The listing builds one solid part. Answer for the finished solid, in the listing's coordinates (mm). Face numbers are marked on the shaded views. A direction names the side the tool comes from. Round coordinates to 2 decimals unless told otherwise and drop trailing zeros. Loops run counter-clockwise (first coordinate to the right, second up) from the corner with the lowest first, then second, coordinate; pieces in that order, holes last. Notation, with made-up numbers: M 48.5,32 L 59.5,32 A11 cw 59.5,51 Z; hole C 76.5,-29.5 d7. An arc over 180 degrees is marked long. Put each result on its own line as item: value. Start each with the question number.
(1) Determine the mould class of the marked faces 1, 2 and 3 for opening direction Z: released by +Z, released by -Z, zero draft, split by the parting line, or undercut.
(2) Straight lines are drawn through the part: line 1 (X direction, y = 10, z = -16); line 2 (X direction, y = 12.5, z = -173.5); line 3 (Z direction, x = -100, y = 23). For each, find the intervals that lie inside material, in ascending order.
(3) Section B-B, the plane z = -173 is taken. Determine the outline of the cut face in (x, y), then the cut area to 3 significant figures.
(4) Which of the six approach directions +Z, -Z, +X, -X, +Y, -Y give full straight-line access (tool end or side, diameter ignored) to the marked faces 4, 5 and 6?
(5) Section C-C, the plane y = 7 is taken. Determine the outline of the cut face in (x, z).
(6) Section A-A, the plane x = 100 is taken. Determine the outline of the cut face in (y, z).
(7) Flat-ended cylindrical pins translate along their axes: P1, Ø5.5, axis at x = 69.5, z = -112, coming from the +Y side; P2, Ø1.5, axis at y = 25.5, z = -79, coming from the +X side; P3, Ø12, axis at y = 23.5, z = -163.5, coming from the -X side; P4, Ø12, axis at x = -54.5, z = -112, coming from the -Y side. Find the tip coordinate at first contact, or state that the pin passes through.
(8) Section D-D, the plane x = 14 is taken. Determine the outline of the cut face in (y, z).
```python
from build123d import *

# Parameters (mm, degrees)
SKETCH1_R                   = 12
BOSS_EXTRUDE1_DEPTH         = 33
FILLET1_R                   = 10
M8_TAPPED_HOLE1_D           = 6.8
M8_TAPPED_HOLE1_DEPTH       = 33
M8_TAPPED_HOLE1_CSINK_D     = 8.05
M8_TAPPED_HOLE1_CSINK_ANGLE = 90
CUT_EXTRUDE1_REACH          = 35


with BuildPart() as part:
    # Sketch1 → Boss-Extrude1 (new body)
    with BuildSketch(Plane(origin=(0, 0, 0), x_dir=(1, 0, 0), z_dir=(0, 1, 0))):
        with BuildLine():
            Line((125, 0), (-125, 0))
            Line((-125, 0), (-125, 148.505102572))
            ThreePointArc((-125, 148.505102572), (-120.023162168, 201.706671295), (-68.377223398, 188))
            Line((-68.377223398, 188), (68.377223398, 188))
            ThreePointArc((68.377223398, 188), (120.023162168, 201.706671295), (125, 148.505102572))
            Line((125, 148.505102572), (125, 0))
        make_face()
        with Locations((-100, 173)):
            Circle(SKETCH1_R, mode=Mode.SUBTRACT)
        with Locations((100, 173)):
            Circle(SKETCH1_R, mode=Mode.SUBTRACT)
    extrude(amount=BOSS_EXTRUDE1_DEPTH)

    # Fillet1
    fillet1_edges = [part.edges().sort_by_distance(p)[0] for p in [
        (-125, 16.5, -148.505102572),
        (-68.377223398, 16.5, -188),
        (68.377223398, 16.5, -188),
        (125, 16.5, -148.505102572),
    ]]
    fillet(fillet1_edges, radius=FILLET1_R)

    # M8 Tapped Hole1
    with Locations(Plane(origin=(0, 33, 0), x_dir=(1, 0, 0), z_dir=(0, 1, 0))):
        with Locations((-69.5, 112), (69.5, 112), (69.5, 16), (-69.5, 16)):
            CounterSinkHole(M8_TAPPED_HOLE1_D / 2, M8_TAPPED_HOLE1_CSINK_D / 2, depth=M8_TAPPED_HOLE1_DEPTH, counter_sink_angle=M8_TAPPED_HOLE1_CSINK_ANGLE)

    # Sketch4 → Cut-Extrude1 (cut, up to next)
    with BuildSketch(Plane(origin=(0, 33, 0), x_dir=(1, 0, 0), z_dir=(0, 1, 0)), mode=Mode.PRIVATE) as cut_extrude1_sk1:
        with BuildLine():
            Line((-41.773055434, 78.602374467), (36.226944566, 78.602374467))
            ThreePointArc((36.226944566, 78.602374467), (51.226944566, 63.602374467), (36.226944566, 48.602374467))
            Line((36.226944566, 48.602374467), (-41.773055434, 48.602374467))
            ThreePointArc((-41.773055434, 48.602374467), (-56.773055434, 63.602374467), (-41.773055434, 78.602374467))
        make_face()
    cut_extrude1_tool1 = extrude(cut_extrude1_sk1.sketch, amount=-CUT_EXTRUDE1_REACH, mode=Mode.PRIVATE) & part.part
    add(cut_extrude1_tool1.solids().sort_by_distance((-2.773055, 33, -63.602374))[0], mode=Mode.SUBTRACT)


solid = part.part
```
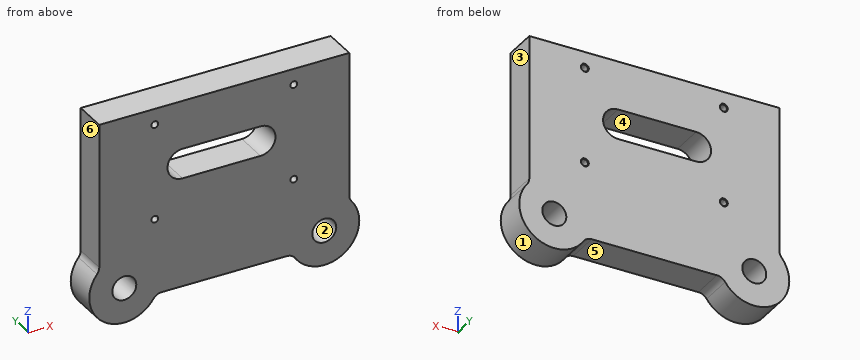
Recorded:
1. face 1: split by the parting line
1. face 2: undercut
1. face 3: zero draft
2. line 1: x = -125 to -72.9, -66.1 to 66.1, 72.9 to 125
2. line 2: x = -135 to -111.99, -88.01 to 88.01, 111.99 to 135
2. line 3: z = -208 to -185, -161 to 0
3. outline: M -135,0 L -112,0 L -112,33 L -135,33 Z; M -88,0 L 88,0 L 88,33 L -88,33 Z; M 112,0 L 135,0 L 135,33 L 112,33 Z
3. area: 7,330 mm²
4. face 4: +Y, -Y
4. face 5: -Z, +Y, -Y
4. face 6: +Z, -X, +Y, -Y
5. outline: M -127.22,-151 A35 ccw long -70.9,-192.44 A10 cw -62.58,-188 L 62.58,-188 A10 cw 70.9,-192.44 A35 ccw long 127.22,-151 A10 cw 125,-144.72 L 125,0 L -125,0 L -125,-144.72 A10 cw Z; hole C -100,-173 d24; hole C -69.5,-112 d6.8; hole C -69.5,-16 d6.8; hole M -41.77,-78.6 L 36.23,-78.6 A15 ccw 36.23,-48.6 L -41.77,-48.6 A15 ccw Z; hole C 69.5,-112 d6.8; hole C 69.5,-16 d6.8; hole C 100,-173 d24
6. outline: M 0,-208 L 33,-208 L 33,-185 L 0,-185 Z; M 0,-161 L 33,-161 L 33,0 L 0,0 Z
7. P1: passes through
7. P2: stops at x = 125
7. P3: stops at x = -134.82
7. P4: stops at y = 0
8. outline: M 0,-188 L 33,-188 L 33,-78.6 L 0,-78.6 Z; M 0,-48.6 L 33,-48.6 L 33,0 L 0,0 Z
